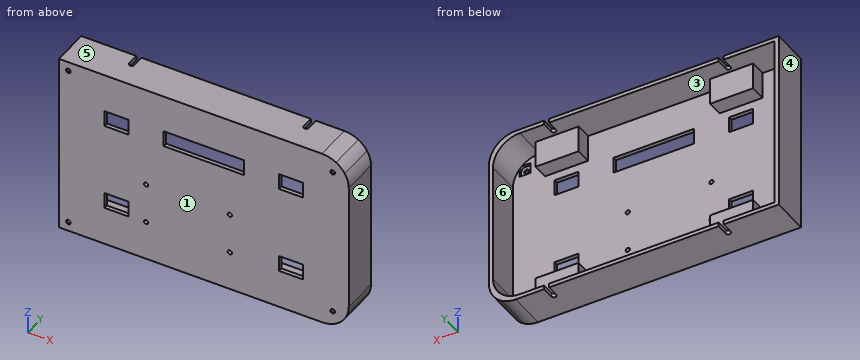
from build123d import *

# Parameters (mm, degrees)
SKETCH1_W                = 210.2
SKETCH1_H                = 130.2
BOSS_EXTRUDE1_DEPTH      = 3
FILLET1_R                = 20
BOSS_EXTRUDE3_DEPTH      = 25
BOSS_EXTRUDE3_DEPTH_BACK = 3
SKETCH2_W                = 216.2
SKETCH2_H                = 136.2
SKETCH2_W_2              = 210.2
SKETCH2_H_2              = 130.2
FILLET2_START            = -1
FILLET2_DEPTH            = 29
FILLET2_2_DEPTH          = 28
SKETCH5_W                = 32.2
SKETCH5_H                = 20
BOSS_EXTRUDE4_DEPTH      = 11.8
MIRROR2_COPY_1_SKETCH_W  = 32.2
MIRROR2_COPY_1_SKETCH_H  = 20
MIRROR2_COPY_1_DEPTH     = 11.8
SKETCH4_W                = 3.7
SKETCH4_H                = 167.196709826
SKETCH4_H_2              = 176.392528866
CUT_EXTRUDE1_DEPTH       = 9
CROQUIS1_R               = 1.75
CORTAR_EXTRUIR1_DEPTH    = 5
CROQUIS2_W               = 18
CROQUIS2_H               = 12
CROQUIS2_W_2             = 60
CORTAR_EXTRUIR2_DEPTH    = 5
CROQUIS3_W               = 8
CROQUIS3_H               = 8
CORTAR_EXTRUIR3_DEPTH    = 2
CORTAR_EXTRUIR4_DEPTH    = 150
CROQUIS5_R               = 1.6
CORTAR_EXTRUIR5_DEPTH    = 10


with BuildPart() as part:
    # Sketch1 → Boss-Extrude1 (new body)
    with BuildSketch(Plane(origin=(0, 0, 0), x_dir=(1, 0, 0), z_dir=(0, 1, 0))):
        Rectangle(SKETCH1_W, SKETCH1_H)
    extrude(amount=BOSS_EXTRUDE1_DEPTH)

    # Fillet1
    fillet1_edges = [part.edges().sort_by_distance(p)[0] for p in [
        (105.1, 1.5, 65.1),
        (105.1, 1.5, -65.1),
    ]]
    fillet(fillet1_edges, radius=FILLET1_R)

    # Sketch2 → Boss-Extrude3 (add, two sides: drawn at the far end of the back side and taken through both)
    with BuildSketch(Plane(origin=(0, 3, 0), x_dir=(1, 0, 0), z_dir=(0, 1, 0)).offset(-BOSS_EXTRUDE3_DEPTH_BACK)):
        Rectangle(SKETCH2_W, SKETCH2_H)
        Rectangle(SKETCH2_W_2, SKETCH2_H_2, mode=Mode.SUBTRACT)
    extrude(amount=BOSS_EXTRUDE3_DEPTH + BOSS_EXTRUDE3_DEPTH_BACK)

    # Fillet2: read off the stored shape, not the designer's step
    # Fillet2 outline → Fillet2 (cut)
    with BuildSketch(Plane(origin=(0, 0, 0), x_dir=(1, 0, 0), z_dir=(0, 1, 0)).offset(FILLET2_START)):
        with BuildLine():
            ThreePointArc((98.635653754, -65.1), (93.577225575, -67.335384062), (88.1, -68.1))
            Line((88.1, -68.1), (108.1, -68.1))
            Line((108.1, -68.1), (108.1, -48.1))
            ThreePointArc((108.1, -48.1), (107.335384062, -53.577225575), (105.1, -58.635653754))
            Line((105.1, -58.635653754), (105.1, -65.1))
            Line((105.1, -65.1), (98.635653754, -65.1))
        make_face()
        with BuildLine():
            ThreePointArc((105.1, 58.635653754), (107.335384062, 53.577225575), (108.1, 48.1))
            Line((108.1, 48.1), (108.1, 68.1))
            Line((108.1, 68.1), (88.1, 68.1))
            ThreePointArc((88.1, 68.1), (93.577225575, 67.335384062), (98.635653754, 65.1))
            Line((98.635653754, 65.1), (105.1, 65.1))
            Line((105.1, 65.1), (105.1, 58.635653754))
        make_face()
    extrude(amount=FILLET2_DEPTH, mode=Mode.SUBTRACT)

    # Fillet2 2 outline → Fillet2 2 (add)
    with BuildSketch(Plane(origin=(0, 0, 0), x_dir=(1, 0, 0), z_dir=(0, 1, 0))):
        with BuildLine():
            Line((85.1, -65.1), (98.635653754, -65.1))
            ThreePointArc((98.635653754, -65.1), (102.242135624, -62.242135624), (105.1, -58.635653754))
            Line((105.1, -58.635653754), (105.1, -45.1))
            ThreePointArc((105.1, -45.1), (99.242135624, -59.242135624), (85.1, -65.1))
        make_face()
        with BuildLine():
            ThreePointArc((85.1, 65.1), (99.242135624, 59.242135624), (105.1, 45.1))
            Line((105.1, 45.1), (105.1, 58.635653754))
            ThreePointArc((105.1, 58.635653754), (102.242135624, 62.242135624), (98.635653754, 65.1))
            Line((98.635653754, 65.1), (85.1, 65.1))
        make_face()
    extrude(amount=FILLET2_2_DEPTH)

    # Sketch5 → Boss-Extrude4 (add)
    with BuildSketch(Plane(origin=(0, 3, 0), x_dir=(1, 0, 0), z_dir=(0, 1, 0))):
        with Locations((-65.1, 55.1)):
            Rectangle(SKETCH5_W, SKETCH5_H)
    boss_extrude4 = extrude(amount=BOSS_EXTRUDE4_DEPTH)

    # Mirror1: Boss-Extrude4 across plane
    add(boss_extrude4.mirror(Plane(origin=(0, 0, 0), x_dir=(0, 0, 1), z_dir=(1, 0, 0))))

    # Mirror2: Boss-Extrude4 across plane
    add(boss_extrude4.mirror(Plane.XY))

    # Mirror2 copy 1 sketch → Mirror2 copy 1 (add)
    with BuildSketch(Plane(origin=(0, 3, 0), x_dir=(-1, 0, 0), z_dir=(0, 1, 0))):
        with Locations((-65.1, 55.1)):
            Rectangle(MIRROR2_COPY_1_SKETCH_W, MIRROR2_COPY_1_SKETCH_H)
    extrude(amount=MIRROR2_COPY_1_DEPTH)

    # Sketch4 → Cut-Extrude1 (cut)
    with BuildSketch(Plane(origin=(0, 28, 0), x_dir=(1, 0, 0), z_dir=(0, 1, 0))):
        with Locations((-65.1, 0)):
            Rectangle(SKETCH4_W, SKETCH4_H)
        with Locations((65.1, 0)):
            Rectangle(SKETCH4_W, SKETCH4_H_2)
    extrude(amount=-CUT_EXTRUDE1_DEPTH, mode=Mode.SUBTRACT)

    # Croquis1 → Cortar-Extruir1 (cut)
    with BuildSketch(Plane.XZ):
        with Locations(Location((-101.1, 61.1, 0), (0, 0, 270))):
            Circle(CROQUIS1_R)
        with Locations(Location((-101.1, -61.1, 0), (0, 0, 270))):
            Circle(CROQUIS1_R)
        with Locations(Location((96.1, 56.1, 0), (0, 0, 270))):
            Circle(CROQUIS1_R)
        with Locations(Location((96.1, -56.1, 0), (0, 0, 270))):
            Circle(CROQUIS1_R)
    extrude(amount=-CORTAR_EXTRUIR1_DEPTH, mode=Mode.SUBTRACT)

    # Croquis2 → Cortar-Extruir2 (cut)
    with BuildSketch(Plane(origin=(0, 3, 0), x_dir=(1, 0, 0), z_dir=(0, 1, 0))):
        with Locations((-65.1, 33.1)):
            Rectangle(CROQUIS2_W, CROQUIS2_H)
        with Locations((-65.1, -33.1)):
            Rectangle(CROQUIS2_W, CROQUIS2_H)
        with Locations((65.1, 33.1)):
            Rectangle(CROQUIS2_W, CROQUIS2_H)
        with Locations((65.1, -33.1)):
            Rectangle(CROQUIS2_W, CROQUIS2_H)
        with Locations((0, -34.1)):
            Rectangle(CROQUIS2_W_2, CROQUIS2_H)
    extrude(amount=-CORTAR_EXTRUIR2_DEPTH, mode=Mode.SUBTRACT)

    # Croquis3 → Cortar-Extruir3 (cut)
    with BuildSketch(Plane(origin=(0, 3, 0), x_dir=(1, 0, 0), z_dir=(0, 1, 0))):
        with BuildLine():
            Line((92.1, 60.1), (96.9, 60.1))
            ThreePointArc((96.9, 60.1), (99.1627417, 59.1627417), (100.1, 56.9))
            Line((100.1, 56.9), (100.1, 52.1))
            Line((100.1, 52.1), (92.1, 52.1))
            Line((92.1, 52.1), (92.1, 60.1))
        make_face()
        with Locations((-101.1, 61.1)):
            Rectangle(CROQUIS3_W, CROQUIS3_H)
        with Locations((-101.1, -61.1)):
            Rectangle(CROQUIS3_W, CROQUIS3_H)
        with BuildLine():
            Line((92.1, -52.1), (100.1, -52.1))
            Line((100.1, -52.1), (100.1, -56.9))
            ThreePointArc((100.1, -56.9), (99.1627417, -59.1627417), (96.9, -60.1))
            Line((96.9, -60.1), (92.1, -60.1))
            Line((92.1, -60.1), (92.1, -52.1))
        make_face()
    extrude(amount=-CORTAR_EXTRUIR3_DEPTH, mode=Mode.SUBTRACT)

    # Croquis4 → Cortar-Extruir4 (cut)
    with BuildSketch(Plane.XY.offset(68.1)):
        with BuildLine():
            Line((-66.95, 19), (-63.25, 19))
            ThreePointArc((-63.25, 19), (-65.1, 17.15), (-66.95, 19))
        make_face()
        with BuildLine():
            Line((66.95, 19), (63.25, 19))
            ThreePointArc((63.25, 19), (65.1, 17.15), (66.95, 19))
        make_face()
    extrude(amount=-CORTAR_EXTRUIR4_DEPTH, mode=Mode.SUBTRACT)

    # Croquis5 → Cortar-Extruir5 (cut)
    with BuildSketch(Plane.XZ):
        with Locations(Location((-43.1, -8.1, 0), (0, 0, 270))):
            Circle(CROQUIS5_R)
        with Locations(Location((-43.1, -38.48, 0), (0, 0, 270))):
            Circle(CROQUIS5_R)
        with Locations(Location((19.36, -8.1, 0), (0, 0, 270))):
            Circle(CROQUIS5_R)
        with Locations(Location((19.36, -38.48, 0), (0, 0, 270))):
            Circle(CROQUIS5_R)
    extrude(amount=-CORTAR_EXTRUIR5_DEPTH, mode=Mode.SUBTRACT)


solid = part.part
Input: part model. Units: mm. Frame: model coordinates. Face numbers are marked on the shaded views. A direction names the side the tool comes from. Give positions to 0.01 mm unless a question says otherwise; leave off trailing zeros. Order: outer loops, then holes, each group sorted by start corner. A loop starts at its lowest first (then second) coordinate and runs counter-clockwise, first axis right, second up.
Q1. Draft query along X for the marked faces 1, 2, 3 and 4. Return one class per face: +X half, -X half, draft (parallel to the pull), parting line (faces both ways), or undercut.
Checked values:
face 1: draft
face 2: +X half
face 3: undercut
face 4: -X half
Q2. Contact query for flat-ended pins moving along their axis: pin 1 Ø1 at (x, y) = (95.5, 1.5) entering from -Z; pin 2 Ø1.6 at (y, z) = (2, 58) entering from +X; pin 3 Ø2.5 at (y, z) = (25, -67) entering from +X. Output: stop coordinate, or through.
Checked values:
pin 1: stops at z = -66.87
pin 2: stops at x = 105.91
pin 3: stops at x = 97.51
Q3. Section A-A on y = 25.25. Output: boundary loops of the cut face in (x, z), and give its area (3 significant figures).
Checked values:
outline: (-108.1, -68.1) - (-66.95, -68.1) - (-66.95, -65.1) - (-105.1, -65.1) - (-105.1, 65.1) - (-66.95, 65.1) - (-66.95, 68.1) - (-108.1, 68.1) - close; (-63.25, -68.1) - (63.25, -68.1) - (63.25, -65.1) - (-63.25, -65.1) - close; (-63.25, 65.1) - (63.25, 65.1) - (63.25, 68.1) - (-63.25, 68.1) - close; (66.95, -68.1) - (88.1, -68.1) arc R20 ccw to (108.1, -48.1) - (108.1, 48.1) arc R20 ccw to (88.1, 68.1) - (66.95, 68.1) - (66.95, 65.1) - (85.1, 65.1) arc R20 cw to (105.1, 45.1) - (105.1, -45.1) arc R20 cw to (85.1, -65.1) - (66.95, -65.1) - close
area: 2,030 mm2
Q4. Section C-C on y = 11. Output: boundary loops of the cut face in (x, z).
Checked values:
outline: (-108.1, -68.1) - (88.1, -68.1) arc R20 ccw to (108.1, -48.1) - (108.1, 48.1) arc R20 ccw to (88.1, 68.1) - (-108.1, 68.1) - close; hole (-105.1, -65.1) - (-81.2, -65.1) - (-81.2, -45.1) - (-49, -45.1) - (-49, -65.1) - (49, -65.1) - (49, -45.1) - (81.2, -45.1) - (81.2, -65.1) - (85.1, -65.1) arc R20 ccw to (105.1, -45.1) - (105.1, 45.1) arc R20 ccw to (85.1, 65.1) - (81.2, 65.1) - (81.2, 45.1) - (49, 45.1) - (49, 65.1) - (-49, 65.1) - (-49, 45.1) - (-81.2, 45.1) - (-81.2, 65.1) - (-105.1, 65.1) - close
Q5. Section D-D on z = -34.5. Output: boundary loops of the cut face in (x, y), and give its area (3 significant figures).
Checked values:
outline: (-108.1, 0) - (-74.1, 0) - (-74.1, 3) - (-105.1, 3) - (-105.1, 28) - (-108.1, 28) - close; (-56.1, 0) - (56.1, 0) - (56.1, 3) - (-56.1, 3) - close; (74.1, 0) - (108.1, 0) - (108.1, 28) - (105.1, 28) - (105.1, 3) - (74.1, 3) - close
area: 691 mm2
Q6. Section B-B on x = -24.5. Output: boundary loops of the cut face in (y, z).
Checked values:
outline: (0, -68.1) - (28, -68.1) - (28, -65.1) - (3, -65.1) - (3, 28.1) - (0, 28.1) - close; (0, 40.1) - (3, 40.1) - (3, 65.1) - (28, 65.1) - (28, 68.1) - (0, 68.1) - close
Q7. Ray query, probe 1 along Z at (x, y) = (-101.1, 0.75); probe 2 along X at (y, z) = (1.85, -38.48); probe 3 along Z at (x, y) = (14.5, 23). Return the intervals inside material, ascending.
Checked values:
probe 1: z = -68.1 to -62.85, -59.35 to 59.35, 62.85 to 68.1
probe 2: x = -108.1 to -74.1, -56.1 to -44.7, -41.5 to 17.76, 20.96 to 56.1, 74.1 to 108.1
probe 3: z = -68.1 to -65.1, 65.1 to 68.1
Q8. Set-up query: the marked faces 5 and 6. Return all of +Z, -Z, +X, -X, +Y, -Y with unobstructed straight access to the full face (end or side cutting, diameter ignored); none if empty.
Checked values:
face 5: +Z, +X, -X, +Y, -Y
face 6: +Y
